Build history of the part. All positions in model axes, mm. Face numbers are marked on the shaded views. A direction names the side the tool comes from. Round coordinates to 2 decimals unless told otherwise and drop trailing zeros. Loops run counter-clockwise (first coordinate to the right, second up) from the corner with the lowest first, then second, coordinate; pieces in that order, holes last. Notation, with made-up numbers: (-13, 48) -> (18, 48) arc R22 ccw to (18, 65) -> close; hole circle Ø7 at (82, 52.5). An arc over 180 degrees is marked (long way). Put each result on its own line as item: value. Start each with the question number.
Item 1: Cut at B-B, the plane z = 16. List the corners of the cut face in (x, y), plus the area to 3 significant figures.
Item 2: Cut at C-C, the plane x = 43. List the corners of the cut face in (y, z).
Item 3: Tool access for the marked faces 1 and 2: list every direction of +Z, -Z, +X, -X, +Y, -Y with a clear straight run to the whole face (end or side of a thin tool).
Item 4: Cut at A-A, the plane y = -9.25. List the corners of the cut face in (x, z), plus the area to 3 significant figures.
Item 5: Drill centre lines: probe 1 along Z at (x, y) = (0, -23.2); probe 2 along Y at (x, z) = (74, 2); probe 3 along X at (y, z) = (-13.5, -30.5). Where is each one in solid material? Low to high. Write a range as [from, to].
Item 6: Cut at D-D, the plane z = -62. List the corners of the cut face in (x, y), plus the area to 3 significant figures.
Item 7: Flat gauge pins, fed straight in: pin 1 Ø12 at (x, y) = (37, -9.5) entering from +Z; pin 2 Ø10 at (y, z) = (-8, 14) entering from +X; pin 3 Ø2 at (y, z) = (-20, -73) entering from -X; pin 4 Ø12 at (y, z) = (-10.5, -10.5) entering from -X. Where does each tip first touch, or does it go through?
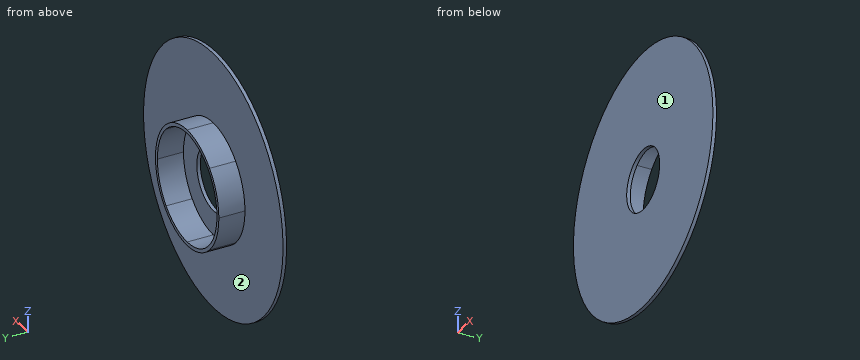
```python
from build123d import *

# Parameters (mm, degrees)
F1_DEPTH = 22
F2_R     = 110
F2_R_2   = 50
F2_R_3   = 47
F3_DEPTH = 3
F4_R     = 26
F5_DEPTH = 3
F6_DEPTH = 25


# Not quite as in the source:
# - a feature names something its author has since deleted; it is built from what else it names


with BuildPart() as f1:
    # F0 (on Front) → F1 (new body)
    with BuildSketch(Plane.XZ):
        with BuildLine():
            Line((48.5, 0), (50, 0))
            ThreePointArc((50, 0), (46.1939766256, 19.1341716183), (35.3553390593, 35.3553390593))
            Line((35.3553390593, 35.3553390593), (34.2946788875, 34.2946788875))
            ThreePointArc((34.2946788875, 34.2946788875), (44.8081573268, 18.5601464697), (48.5, 0))
        make_face()
        with BuildLine():
            ThreePointArc((35.3553390593, -35.3553390593), (46.1939766256, -19.1341716183), (50, 0))
            Line((50, 0), (48.5, 0))
            ThreePointArc((48.5, 0), (44.8081573268, -18.5601464697), (34.2946788875, -34.2946788875))
            Line((34.2946788875, -34.2946788875), (35.3553390593, -35.3553390593))
        make_face()
        with BuildLine():
            Line((34.2946788875, 34.2946788875), (35.3553390593, 35.3553390593))
            ThreePointArc((35.3553390593, 35.3553390593), (19.1341716183, 46.1939766256), (0, 50))
            Line((0, 50), (0, 48.5))
            ThreePointArc((0, 48.5), (18.5601464697, 44.8081573268), (34.2946788875, 34.2946788875))
        make_face()
        with BuildLine():
            ThreePointArc((0, -50), (19.1341716183, -46.1939766256), (35.3553390593, -35.3553390593))
            Line((35.3553390593, -35.3553390593), (34.2946788875, -34.2946788875))
            ThreePointArc((34.2946788875, -34.2946788875), (18.5601464697, -44.8081573268), (0, -48.5))
            Line((0, -48.5), (0, -50))
        make_face()
        with BuildLine():
            Line((47, 0), (48.5, 0))
            ThreePointArc((48.5, 0), (44.8081573268, 18.5601464697), (34.2946788875, 34.2946788875))
            Line((34.2946788875, 34.2946788875), (33.2340187158, 33.2340187158))
            ThreePointArc((33.2340187158, 33.2340187158), (43.422338028, 17.9861213212), (47, 0))
        make_face()
        with BuildLine():
            ThreePointArc((34.2946788875, -34.2946788875), (44.8081573268, -18.5601464697), (48.5, 0))
            Line((48.5, 0), (47, 0))
            ThreePointArc((47, 0), (43.422338028, -17.9861213212), (33.2340187158, -33.2340187158))
            Line((33.2340187158, -33.2340187158), (34.2946788875, -34.2946788875))
        make_face()
        with BuildLine():
            Line((0, 48.5), (0, 50))
            ThreePointArc((0, 50), (-19.1341716183, 46.1939766256), (-35.3553390593, 35.3553390593))
            Line((-35.3553390593, 35.3553390593), (-34.2946788875, 34.2946788875))
            ThreePointArc((-34.2946788875, 34.2946788875), (-18.5601464697, 44.8081573268), (0, 48.5))
        make_face()
        with BuildLine():
            Line((33.2340187158, 33.2340187158), (34.2946788875, 34.2946788875))
            ThreePointArc((34.2946788875, 34.2946788875), (18.5601464697, 44.8081573268), (0, 48.5))
            Line((0, 48.5), (0, 47))
            ThreePointArc((0, 47), (17.9861213212, 43.422338028), (33.2340187158, 33.2340187158))
        make_face()
        with BuildLine():
            ThreePointArc((-35.3553390593, -35.3553390593), (-19.1341716183, -46.1939766256), (0, -50))
            Line((0, -50), (0, -48.5))
            ThreePointArc((0, -48.5), (-18.5601464697, -44.8081573268), (-34.2946788875, -34.2946788875))
            Line((-34.2946788875, -34.2946788875), (-35.3553390593, -35.3553390593))
        make_face()
        with BuildLine():
            ThreePointArc((0, -48.5), (18.5601464697, -44.8081573268), (34.2946788875, -34.2946788875))
            Line((34.2946788875, -34.2946788875), (33.2340187158, -33.2340187158))
            ThreePointArc((33.2340187158, -33.2340187158), (17.9861213212, -43.422338028), (0, -47))
            Line((0, -47), (0, -48.5))
        make_face()
        with BuildLine():
            Line((-34.2946788875, 34.2946788875), (-35.3553390593, 35.3553390593))
            ThreePointArc((-35.3553390593, 35.3553390593), (-46.1939766256, 19.1341716183), (-50, 0))
            Line((-50, 0), (-48.5, 0))
            ThreePointArc((-48.5, 0), (-44.8081573268, 18.5601464697), (-34.2946788875, 34.2946788875))
        make_face()
        with BuildLine():
            Line((0, 47), (0, 48.5))
            ThreePointArc((0, 48.5), (-18.5601464697, 44.8081573268), (-34.2946788875, 34.2946788875))
            Line((-34.2946788875, 34.2946788875), (-33.2340187158, 33.2340187158))
            ThreePointArc((-33.2340187158, 33.2340187158), (-17.9861213212, 43.422338028), (0, 47))
        make_face()
        with BuildLine():
            ThreePointArc((-50, 0), (-46.1939766256, -19.1341716183), (-35.3553390593, -35.3553390593))
            Line((-35.3553390593, -35.3553390593), (-34.2946788875, -34.2946788875))
            ThreePointArc((-34.2946788875, -34.2946788875), (-44.8081573268, -18.5601464697), (-48.5, 0))
            Line((-48.5, 0), (-50, 0))
        make_face()
        with BuildLine():
            ThreePointArc((-34.2946788875, -34.2946788875), (-18.5601464697, -44.8081573268), (0, -48.5))
            Line((0, -48.5), (0, -47))
            ThreePointArc((0, -47), (-17.9861213212, -43.422338028), (-33.2340187158, -33.2340187158))
            Line((-33.2340187158, -33.2340187158), (-34.2946788875, -34.2946788875))
        make_face()
        with BuildLine():
            Line((-33.2340187158, 33.2340187158), (-34.2946788875, 34.2946788875))
            ThreePointArc((-34.2946788875, 34.2946788875), (-44.8081573268, 18.5601464697), (-48.5, 0))
            Line((-48.5, 0), (-47, 0))
            ThreePointArc((-47, 0), (-43.422338028, 17.9861213212), (-33.2340187158, 33.2340187158))
        make_face()
        with BuildLine():
            ThreePointArc((-48.5, 0), (-44.8081573268, -18.5601464697), (-34.2946788875, -34.2946788875))
            Line((-34.2946788875, -34.2946788875), (-33.2340187158, -33.2340187158))
            ThreePointArc((-33.2340187158, -33.2340187158), (-43.422338028, -17.9861213212), (-47, 0))
            Line((-47, 0), (-48.5, 0))
        make_face()
    extrude(amount=F1_DEPTH)

    # F2 (on face) → F3 (join)
    with BuildSketch(Plane.XZ.offset(22)):
        Circle(F2_R)
        Circle(F2_R_2, mode=Mode.SUBTRACT)
        Circle(F2_R_2)
        Circle(F2_R_3, mode=Mode.SUBTRACT)
        Circle(F2_R_3)
    extrude(amount=F3_DEPTH)

    # F4 (on face) → F5 (cut, through all)
    with BuildSketch(Plane.XZ.offset(25)):
        Circle(F4_R)
    extrude(amount=-F5_DEPTH, mode=Mode.SUBTRACT)

    # F0 (on Front) → F6 (join)
    with BuildSketch(Plane.XZ):
        with BuildLine():
            Line((48.5, 0), (50, 0))
            ThreePointArc((50, 0), (46.1939766256, 19.1341716183), (35.3553390593, 35.3553390593))
            Line((35.3553390593, 35.3553390593), (34.2946788875, 34.2946788875))
            ThreePointArc((34.2946788875, 34.2946788875), (44.8081573268, 18.5601464697), (48.5, 0))
        make_face()
        with BuildLine():
            ThreePointArc((35.3553390593, -35.3553390593), (46.1939766256, -19.1341716183), (50, 0))
            Line((50, 0), (48.5, 0))
            ThreePointArc((48.5, 0), (44.8081573268, -18.5601464697), (34.2946788875, -34.2946788875))
            Line((34.2946788875, -34.2946788875), (35.3553390593, -35.3553390593))
        make_face()
        with BuildLine():
            Line((34.2946788875, 34.2946788875), (35.3553390593, 35.3553390593))
            ThreePointArc((35.3553390593, 35.3553390593), (19.1341716183, 46.1939766256), (0, 50))
            Line((0, 50), (0, 48.5))
            ThreePointArc((0, 48.5), (18.5601464697, 44.8081573268), (34.2946788875, 34.2946788875))
        make_face()
        with BuildLine():
            ThreePointArc((0, -50), (19.1341716183, -46.1939766256), (35.3553390593, -35.3553390593))
            Line((35.3553390593, -35.3553390593), (34.2946788875, -34.2946788875))
            ThreePointArc((34.2946788875, -34.2946788875), (18.5601464697, -44.8081573268), (0, -48.5))
            Line((0, -48.5), (0, -50))
        make_face()
        with BuildLine():
            Line((0, 48.5), (0, 50))
            ThreePointArc((0, 50), (-19.1341716183, 46.1939766256), (-35.3553390593, 35.3553390593))
            Line((-35.3553390593, 35.3553390593), (-34.2946788875, 34.2946788875))
            ThreePointArc((-34.2946788875, 34.2946788875), (-18.5601464697, 44.8081573268), (0, 48.5))
        make_face()
        with BuildLine():
            ThreePointArc((-35.3553390593, -35.3553390593), (-19.1341716183, -46.1939766256), (0, -50))
            Line((0, -50), (0, -48.5))
            ThreePointArc((0, -48.5), (-18.5601464697, -44.8081573268), (-34.2946788875, -34.2946788875))
            Line((-34.2946788875, -34.2946788875), (-35.3553390593, -35.3553390593))
        make_face()
        with BuildLine():
            Line((-34.2946788875, 34.2946788875), (-35.3553390593, 35.3553390593))
            ThreePointArc((-35.3553390593, 35.3553390593), (-46.1939766256, 19.1341716183), (-50, 0))
            Line((-50, 0), (-48.5, 0))
            ThreePointArc((-48.5, 0), (-44.8081573268, 18.5601464697), (-34.2946788875, 34.2946788875))
        make_face()
        with BuildLine():
            ThreePointArc((-50, 0), (-46.1939766256, -19.1341716183), (-35.3553390593, -35.3553390593))
            Line((-35.3553390593, -35.3553390593), (-34.2946788875, -34.2946788875))
            ThreePointArc((-34.2946788875, -34.2946788875), (-44.8081573268, -18.5601464697), (-48.5, 0))
            Line((-48.5, 0), (-50, 0))
        make_face()
    extrude(amount=F6_DEPTH)


solid = f1.part
```
Reply:
1. outline: (-108.83, -25) -> (-20.49, -25) -> (-20.49, -22) -> (-44.19, -22) -> (-44.19, 0) -> (-47.37, 0) -> (-47.37, -22) -> (-108.83, -22) -> close; (20.49, -25) -> (108.83, -25) -> (108.83, -22) -> (47.37, -22) -> (47.37, 0) -> (44.19, 0) -> (44.19, -22) -> (20.49, -22) -> close
1. area: 670 mm^2
2. outline: (-25, -101.25) -> (-22, -101.25) -> (-22, -25.51) -> (0, -25.51) -> (0, -18.97) -> (-22, -18.97) -> (-22, 18.97) -> (0, 18.97) -> (0, 25.51) -> (-22, 25.51) -> (-22, 101.25) -> (-25, 101.25) -> close
3. face 1: +Z, -Z, +X, -X, -Y
3. face 2: +Y
4. outline: circle Ø100 at (0, 0); hole circle Ø94 at (0, 0)
4. area: 914 mm^2
5. probe 1: z = [-110, -26], [26, 110]
5. probe 2: y = [-25, -22]
5. probe 3: x = [-39.62, -35.76], [35.76, 39.62]
6. outline: (-90.86, -25) -> (90.86, -25) -> (90.86, -22) -> (-90.86, -22) -> close
6. area: 545 mm^2
7. pin 1: stops at z = 39.23
7. pin 2: stops at x = 49.18
7. pin 3: passes through
7. pin 4: stops at x = -49.8
